from build123d import *

# Parameters (mm, degrees)
BOSS_EXTRUDE1_DEPTH = 38
BOSS_EXTRUDE3_DEPTH = 30
CUT_EXTRUDE2_DEPTH  = 61
CUT_EXTRUDE1_DEPTH  = 61


with BuildPart() as part:
    # Sketch1 → Boss-Extrude1 (new body)
    with BuildSketch(Plane.XY):
        with BuildLine():
            Line((-16.024694199, 26.673676157), (3.975305801, 26.673676157))
            Line((3.975305801, 26.673676157), (3.975305801, -3.326323843))
            Line((3.975305801, -3.326323843), (-16.024694199, -3.326323843))
            ThreePointArc((-16.024694199, -3.326323843), (-31.024694199, 11.673676157), (-16.024694199, 26.673676157))
        make_face()
    extrude(amount=BOSS_EXTRUDE1_DEPTH)

    # Sketch2 → Boss-Extrude3 (add)
    with BuildSketch(Plane.XZ.offset(3.326323843)):
        Polygon((3.975305801, 38), (3.975305801, 10.402664479), (28.894576723, 41.635004813), (20.3703899, 49.791936592), align=None)
    extrude(amount=-BOSS_EXTRUDE3_DEPTH)

    # Sketch4 → Cut-Extrude2 (cut)
    with BuildSketch(Plane.XZ.offset(3.326323843)):
        with BuildLine():
            Line((-6.024694199, 0), (8.586429147, -30.750559355))
            Line((8.586429147, -30.750559355), (53.639483602, 0))
            Line((53.639483602, 0), (3.975305801, 10.402664479))
            ThreePointArc((3.975305801, 10.402664479), (-0.784676233, 4.970604847), (-6.024694199, 0))
        make_face()
    extrude(amount=-CUT_EXTRUDE2_DEPTH, mode=Mode.SUBTRACT)

    # Sketch3 → Cut-Extrude1 (cut)
    with BuildSketch(Plane(origin=(0, 0, 0), x_dir=(-1, 0, 0), z_dir=(0, 0, -1))):
        with BuildLine():
            Line((-14.471237169, 14.471119338), (-28.894576723, 18.506537052))
            Line((-28.894576723, 18.506537052), (-57.421554234, 26.725830047))
            Line((-57.421554234, 26.725830047), (-3.301256906, -44.718260526))
            Line((-3.301256906, -44.718260526), (16.024694199, -3.326323843))
            ThreePointArc((16.024694199, -3.326323843), (7.12126065, -1.239294), (0.072764407, 4.586984677))
            ThreePointArc((0.072764407, 4.586984677), (-6.391299116, 10.717890613), (-14.471237169, 14.471119338))
        make_face()
    extrude(amount=-CUT_EXTRUDE1_DEPTH, mode=Mode.SUBTRACT)


solid = part.part
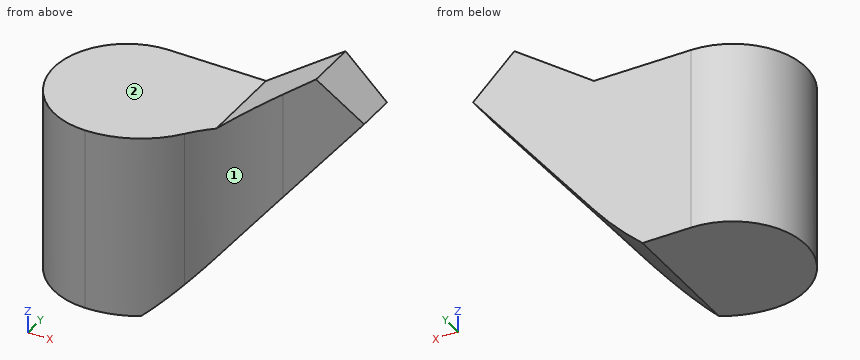
Verification items for the finished model (mm, model axes). Face numbers are marked on the shaded views. A direction names the side the tool comes from. Give positions to 0.01 mm unless a question says otherwise; leave off trailing zeros. Write each loop counter-clockwise with the first axis right and the second up, starting at its lowest first coordinate (ties: lowest second). Pieces come first, ordered by that corner, then holes. Notation, with made-up numbers: M 17.25,8.25 L 70.25,8.25 A13 cw 70.25,29.25 Z; hole C 12.5,-7.5 d2. An arc over 180 degrees is marked long. Put each result on its own line as item: value. Start each with the question number.
1. Set-up check for the marked faces 1 and 2: record each of +Z, -Z, +X, -X, +Y, -Y from which the full face is reachable in a straight line by a thin tool's end or side.
2. Section check B-B (y = 21). Record the cut outline in (x, z) (3 decimals), and give its area (3 significant figures).
3. Go/stop test with flat-tipped pins: pin 1 Ø3 at (x, z) = (-20, 40) entering from -Y; pin 2 Ø4 at (x, y) = (1.5, 21) entering from +Z; pin 3 Ø12 at (x, y) = (2, 8.5) entering from +Z; pin 4 Ø1.5 at (y, z) = (2, 14.5) entering from +X. Record where each tip stops, or that it passes through.
4. Section check C-C (x = 19). Record the cut outline in (y, z), and give its area (3 significant figures).
5. Section check D-D (z = 37). Record the cut outline in (x, y), and give its area (3 significant figures).
6. Section check A-A (z = 17). Record the cut outline in (x, y), and give its area (3 significant figures).
7. Scan lines: line 1 along Y through (x, z) = (-5, 34); line 2 along Z through (x, y) = (-25.5, 12); line 3 along X through (y, z) = (21, 47). Record each from-to range of solid material in increasing order. Write a range as [from, to].
Answer list:
1. face 1: +Z, -Z, +X, -Y
1. face 2: +Z, -X, +Y, -Y
2. outline: M -27.773,0 L -6.025,0 A78.341 ccw 3.975,10.403 L 28.895,41.635 L 20.37,49.792 L 3.975,38 L -27.773,38 Z
2. area: 1,620 mm2
3. pin 1: through
3. pin 2: z = 38
3. pin 3: z = 40.39
3. pin 4: x = -1.65
4. outline: M 15.74,29.23 L 26.67,29.23 L 26.67,48.81 L 15.74,48.81 Z
4. area: 214 mm2
5. outline: M -16.02,-3.33 A20.03 ccw -0.07,4.59 A27.61 cw 14.47,14.47 L 25.2,17.47 L 25.2,26.67 L -16.02,26.67 A15 ccw Z
5. area: 1,140 mm2
6. outline: M -16.02,-3.33 A20.03 ccw -0.07,4.59 A27.61 cw 9.24,12.41 L 9.24,26.67 L -16.02,26.67 A15 ccw Z
6. area: 958 mm2
7. line 1: [-0.02, 26.67]
7. line 2: [0, 38]
7. line 3: [16.49, 23.29]
